Source: CAD feature listing. Evaluate the final solid. Frame: model axes, mm. Face numbers are marked on the shaded views. A direction names the side the tool comes from. Give positions to 0.01 mm unless a question says otherwise; leave off trailing zeros. Order: outer loops, then holes, each group sorted by start corner. A loop starts at its lowest first (then second) coordinate and runs counter-clockwise, first axis right, second up.
1) Section C-C, the plane x = -15.5. Return loops of the section in (y, z), plus the area to 3 significant figures.
2) Section A-A, the plane x = -41.5. Return loops of the section in (y, z), plus the area to 3 significant figures.
3) Section D-D, the plane y = -12.5. Return loops of the section in (x, z), plus the area to 3 significant figures.
4) Section B-B, the plane y = 1. Return loops of the section in (x, z).
5) Draft query along Y for the marked faces 4, 5 and 6. Return one class per face: released by +Y, released by -Y, zero draft, split by the parting line, or undercut.
6) First-contact query: P1, Ø3, axis at x = 14.5, y = -6, coming from the +Z side; P2, Ø1.5, axis at y = 0, z = -4.5, coming from the -X side; P3, Ø2.5, axis at x = -45, y = 15, coming from the +Z side; P4, Ø7.5, axis at x = -46, y = -3, coming from the -Z side. Flat tips, straight axial feed; report the tip coordinate or a pass-through.
7) Material intervals for line 1 (Y direction, x = -45, z = 0.1); line 2 (X direction, y = 6, z = 1); line 3 (X direction, y = 4.5, z = -5), sorted ascending.
8) Access query for the marked faces 1, 2 and 3. Directions: +Z, -Z, +X, -X, +Y, -Y. A direction counts if a zero-diameter tool reaches every point of the face in a straight line with its end or side. Return the directions, or none.
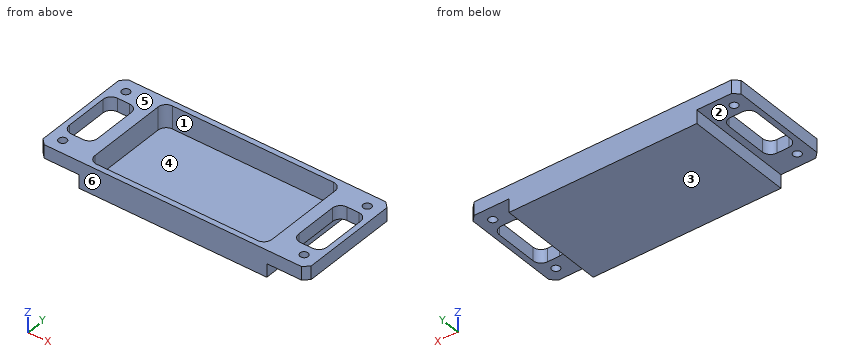
```python
from build123d import *

# Parameters (mm, degrees)
AUFSATZ_LINEAR_AUSTRAGEN1_DEPTH      = 2.5
AUFSATZ_LINEAR_AUSTRAGEN1_DEPTH_BACK = 2.5
SKIZZE1_W                            = 100
SKIZZE1_H                            = 40
SCHNITT_LINEAR_AUSTRAGEN1_DEPTH      = 54.909646632
SCHNITT_LINEAR_AUSTRAGEN1_DEPTH_BACK = 54.909646632
SKIZZE2_R                            = 1.5
SCHNITT_LINEAR_AUSTRAGEN2_DEPTH      = 54.909646632
SCHNITT_LINEAR_AUSTRAGEN2_DEPTH_BACK = 54.909646632
SKIZZE7_W                            = 70
SKIZZE7_H                            = 40
AUFSATZ_LINEAR_AUSTRAGEN3_DEPTH      = 5
SCHNITT_LINEAR_AUSTRAGEN6_DEPTH      = 8.5
FASE1_SIZE                           = 2


with BuildPart() as part:
    # Skizze1 → Aufsatz-Linear austragen1 (new, two sides: drawn at the far end of the back side and taken through both)
    with BuildSketch(Plane.XY.offset(-AUFSATZ_LINEAR_AUSTRAGEN1_DEPTH_BACK)):
        Rectangle(SKIZZE1_W, SKIZZE1_H)
    extrude(amount=AUFSATZ_LINEAR_AUSTRAGEN1_DEPTH + AUFSATZ_LINEAR_AUSTRAGEN1_DEPTH_BACK)

    # Skizze2 → Schnitt-Linear austragen1 (cut, two sides: drawn at the far end of the back side and taken through both)
    with BuildSketch(Plane.XY.offset(-SCHNITT_LINEAR_AUSTRAGEN1_DEPTH_BACK)):
        with Locations((-45, 15)):
            Circle(SKIZZE2_R)
        with Locations(Location((-45, -15, 0), (0, 0, 180))):
            Circle(SKIZZE2_R)
        with Locations((45, -15)):
            Circle(SKIZZE2_R)
        with Locations(Location((45, 15, 0), (0, 0, 180))):
            Circle(SKIZZE2_R)
    extrude(amount=SCHNITT_LINEAR_AUSTRAGEN1_DEPTH + SCHNITT_LINEAR_AUSTRAGEN1_DEPTH_BACK, mode=Mode.SUBTRACT)

    # Skizze4 → Schnitt-Linear austragen2 (cut, two sides: drawn at the far end of the back side and taken through both)
    with BuildSketch(Plane.XY.offset(-SCHNITT_LINEAR_AUSTRAGEN2_DEPTH_BACK)):
        with BuildLine():
            Line((-48, -8), (-48, 8))
            ThreePointArc((-48, 8), (-47.121320344, 10.121320344), (-45, 11))
            Line((-45, 11), (-40.5, 11))
            ThreePointArc((-40.5, 11), (-38.378679656, 10.121320344), (-37.5, 8))
            Line((-37.5, 8), (-37.5, -8))
            ThreePointArc((-37.5, -8), (-38.378679656, -10.121320344), (-40.5, -11))
            Line((-40.5, -11), (-45, -11))
            ThreePointArc((-45, -11), (-47.121320344, -10.121320344), (-48, -8))
        make_face()
        with BuildLine():
            Line((45, -11), (40.5, -11))
            ThreePointArc((40.5, -11), (38.378679656, -10.121320344), (37.5, -8))
            Line((37.5, -8), (37.5, 8))
            ThreePointArc((37.5, 8), (38.378679656, 10.121320344), (40.5, 11))
            Line((40.5, 11), (45, 11))
            ThreePointArc((45, 11), (47.121320344, 10.121320344), (48, 8))
            Line((48, 8), (48, -8))
            ThreePointArc((48, -8), (47.121320344, -10.121320344), (45, -11))
        make_face()
    extrude(amount=SCHNITT_LINEAR_AUSTRAGEN2_DEPTH + SCHNITT_LINEAR_AUSTRAGEN2_DEPTH_BACK, mode=Mode.SUBTRACT)

    # Skizze7 → Aufsatz-Linear austragen3 (add)
    with BuildSketch(Plane(origin=(0, 0, -2.5), x_dir=(-1, 0, 0), z_dir=(0, 0, -1))):
        Rectangle(SKIZZE7_W, SKIZZE7_H)
    extrude(amount=AUFSATZ_LINEAR_AUSTRAGEN3_DEPTH)

    # Skizze8 → Schnitt-Linear austragen6 (cut)
    with BuildSketch(Plane.XY.offset(2.5)):
        with BuildLine():
            Line((33, -15), (33, 15))
            ThreePointArc((33, 15), (32.121320344, 17.121320344), (30, 18))
            Line((30, 18), (-30, 18))
            ThreePointArc((-30, 18), (-32.121320344, 17.121320344), (-33, 15))
            Line((-33, 15), (-33, -15))
            ThreePointArc((-33, -15), (-32.121320344, -17.121320344), (-30, -18))
            Line((-30, -18), (30, -18))
            ThreePointArc((30, -18), (32.121320344, -17.121320344), (33, -15))
        make_face()
    extrude(amount=-SCHNITT_LINEAR_AUSTRAGEN6_DEPTH, mode=Mode.SUBTRACT)

    # Fase1
    fase1_edges = [part.edges().sort_by_distance(p)[0] for p in [
        (50, 20, 0),
        (50, -20, 0),
        (-50, -20, 0),
        (-50, 20, 0),
    ]]
    chamfer(fase1_edges, length=FASE1_SIZE)


solid = part.part
```
From the geometry:
1. outline: (-20, -7.5) - (20, -7.5) - (20, 2.5) - (18, 2.5) - (18, -6) - (-18, -6) - (-18, 2.5) - (-20, 2.5) - close
1. area: 94.0 mm2
2. outline: (-20, -2.5) - (-11, -2.5) - (-11, 2.5) - (-20, 2.5) - close; (11, -2.5) - (20, -2.5) - (20, 2.5) - (11, 2.5) - close
2. area: 90.0 mm2
3. outline: (-50, -2.5) - (-35, -2.5) - (-35, -7.5) - (35, -7.5) - (35, -2.5) - (50, -2.5) - (50, 2.5) - (33, 2.5) - (33, -6) - (-33, -6) - (-33, 2.5) - (-50, 2.5) - close
3. area: 289 mm2
4. outline: (-50, -2.5) - (-48, -2.5) - (-48, 2.5) - (-50, 2.5) - close; (-37.5, -2.5) - (-35, -2.5) - (-35, -7.5) - (35, -7.5) - (35, -2.5) - (37.5, -2.5) - (37.5, 2.5) - (33, 2.5) - (33, -6) - (-33, -6) - (-33, 2.5) - (-37.5, 2.5) - close; (48, -2.5) - (50, -2.5) - (50, 2.5) - (48, 2.5) - close
5. face 4: undercut
5. face 5: zero draft
5. face 6: released by -Y
6. P1: stops at z = -6
6. P2: stops at x = -35
6. P3: passes through
6. P4: stops at z = -2.5
7. line 1: y = -20 to -16.5, -13.5 to -11, 11 to 13.5, 16.5 to 20
7. line 2: x = -50 to -48, -37.5 to -33, 33 to 37.5, 48 to 50
7. line 3: x = -35 to -33, 33 to 35
8. face 1: +Z
8. face 2: -Z, -X, +Y, -Y
8. face 3: -Z, +X, -X, +Y, -Y
